from build123d import *

# Parameters (mm, degrees)
F0_W     = 63.5
F0_H     = 63.5
F1_DEPTH = 3.175
F2_R     = 25.4
F3_DEPTH = 25.4
F4_R     = 6.35


with BuildPart() as f1:
    # F0 (on Top) → F1 (new body)
    with BuildSketch(Plane.XY):
        Rectangle(F0_W, F0_H)
    extrude(amount=F1_DEPTH)

    # F2 (on face) → F3 (join)
    with BuildSketch(Plane.XY.offset(3.175)):
        Circle(F2_R)
    extrude(amount=F3_DEPTH)

    # F4
    f4_edges = [f1.edges().sort_by_distance(p)[0] for p in [
        (-25.4, 0, 28.575),
    ]]
    fillet(f4_edges, radius=F4_R)


solid = f1.part
Geometry: final body of the model. Coordinates: model frame, mm. A direction names the side the tool comes from. Give positions to 0.01 mm unless a question says otherwise; leave off trailing zeros. Write each loop counter-clockwise with the first axis right and the second up, starting at its lowest first coordinate (ties: lowest second). Pieces come first, ordered by that corner, then holes. Notation, with made-up numbers: M 87,-28.5 L 109,-28.5 A23 ccw 109,-11.5 Z; hole C 73,76.25 d7. An arc over 180 degrees is marked long. Answer in a Markdown table with one row per item. Add a question column.
(1) Section A-A on x = 0. Return loops of the section in (y, z) (3 decimals).
(2) Section C-C on z = 17. Return loops of the section in (x, y).
(3) Ray query, line 1 (Z direction, x = -25.5, y = 28.5) (3 decimals); line 2 (X direction, y = 19.5, z = 21); line 3 (Y direction, x = 14.5, z = 3.25). Return the intervals inside material, ascending.
(4) Section D-D on x = -27. Return loops of the section in (y, z) (3 decimals), and give its area (3 significant figures).
(5) Reachability of faces 1 (the flat face through (0, 0, 28.575)), 2 (the cylindrical face through (-5.506, -24.796, 12.567)) from +Z, -Z, +X, -X, +Y, -Y: full face, straight path, thin tool, end or side. Return the list, or none.
(6) First-contact query: pin 1 (4 mm diameter, centred on x = 23, z = 10.5, fed in from +Y); pin 2 (10 mm diameter, centred on x = 4, z = 15, fed in from +Y); pin 3 (5 mm diameter, centred on x = -10, z = 25, fed in from -Y). Flat tips, straight axial feed; report the tip coordinate or a pass-through.
Result set:
| question | item | result |
|---|---|---|
| 1 | outline | M -31.75,0 L 31.75,0 L 31.75,3.175 L 25.4,3.175 L 25.4,22.225 A6.35 ccw 19.05,28.575 L -19.05,28.575 A6.35 ccw -25.4,22.225 L -25.4,3.175 L -31.75,3.175 Z |
| 2 | outline | C 0,0 d50.8 |
| 3 | line 1 | z = 0 to 3.175 |
| 3 | line 2 | x = -16.28 to 16.28 |
| 3 | line 3 | y = -20.85 to 20.85 |
| 4 | outline | M -31.75,0 L 31.75,0 L 31.75,3.175 L -31.75,3.175 Z |
| 4 | area | 202 mm^2 |
| 5 | face 1 | +Z, +X, -X, +Y, -Y |
| 5 | face 2 | +Z |
| 6 | pin 1 | stops at y = 14.29 |
| 6 | pin 2 | stops at y = 25.4 |
| 6 | pin 3 | stops at y = -23.97 |
